Verification items for the finished model (mm, model axes). Face numbers are marked on the shaded views. A direction names the side the tool comes from. Coordinates: 2 decimals unless noted, no trailing zeros. Write each loop counter-clockwise with the first axis right and the second up, starting at its lowest first coordinate (ties: lowest second). Pieces come first, ordered by that corner, then holes. Notation, with made-up numbers: (33.5, -1.5) - (75.5, -1.5) arc R22 cw to (75.5, 19.5) - close; hole circle Ø2 at (57, 58.25). An arc over 180 degrees is marked (long way). Answer as CSV lines item,"result". Start each with the question number.
```python
from build123d import *

# Parameters (mm, degrees)
ESQUISSE1_W              = 8.5
ESQUISSE1_H              = 72
ESQUISSE1_R              = 2.1
BOSS_EXTRU_1_DEPTH       = 17.5
ENL_V_START              = -3
ENL_V_MAT_EXTRU_4_DEPTH  = 3.5
ESQUISSE7_R              = 2.1
BOSS_EXTRU_3_DEPTH       = 7
ESQUISSE3_W              = 8.5
ESQUISSE3_H              = 4
ENL_V_MAT_EXTRU_3_DEPTH  = 19
BOSS_EXTRU_2_START       = -7
BOSS_EXTRU_2_DEPTH       = 12
ESQUISSE8_W              = 8.5
ESQUISSE8_H              = 7
BOSS_EXTRU_4_DEPTH       = 4
ESQUISSE9_R              = 1.6
ENL_V_MAT_EXTRU_5_DEPTH  = 5
ENL_V_START_2            = -4
ESQUISSE10_R             = 1.6
ENL_V_MAT_EXTRU_6_DEPTH  = 2.6
ESQUISSE11_R             = 1.6
ENL_V_MAT_EXTRU_7_DEPTH  = 1.6
ESQUISSE14_W             = 2.5
ESQUISSE14_H             = 10
ENL_V_MAT_EXTRU_9_DEPTH  = 17.6
CHANFREIN1_SIZE          = 0.5
ESQUISSE15_W             = 8.5
ESQUISSE15_H             = 15
ESQUISSE15_W_2           = 2.6
ESQUISSE15_H_2           = 5.7
ESQUISSE15_W_3           = 2.5
ESQUISSE15_H_3           = 10
ENL_V_MAT_EXTRU_10_DEPTH = 10
CHANFREIN2_SIZE          = 9


with BuildPart() as part:
    # Esquisse1 → Boss.-Extru.1 (new body)
    with BuildSketch(Plane.XY):
        with Locations((4.25, 36)):
            Rectangle(ESQUISSE1_W, ESQUISSE1_H)
        with Locations((4, 20.5)):
            Circle(ESQUISSE1_R, mode=Mode.SUBTRACT)
        with Locations((4, 51.5)):
            Circle(ESQUISSE1_R, mode=Mode.SUBTRACT)
    extrude(amount=BOSS_EXTRU_1_DEPTH)

    # Esquisse6 → Enlèv. mat.-Extru.4 (cut)
    with BuildSketch(Plane.XY.offset(17.5).offset(ENL_V_START)):
        Polygon((7.55, 22.549593456), (4, 24.599186911), (0.45, 22.549593456), (0.45, 18.450406544), (4, 16.400813089), (7.55, 18.450406544), align=None)
        Polygon((8.5, 24.599186911), (4, 24.599186911), (7.55, 22.549593456), (7.55, 18.450406544), (4, 16.400813089), (8.5, 16.400813089), align=None)
    enl_v_mat_extru_4 = extrude(amount=-ENL_V_MAT_EXTRU_4_DEPTH, mode=Mode.SUBTRACT)

    # Esquisse7 → Boss.-Extru.3 (add)
    with BuildSketch(Plane(origin=(0, 0, 0), x_dir=(-1, 0, 0), z_dir=(0, 0, -1))):
        with Locations((-4, 20.5)):
            Circle(ESQUISSE7_R)
    boss_extru_3 = extrude(amount=-BOSS_EXTRU_3_DEPTH)

    # Esquisse3 → Enlèv. mat.-Extru.3 (cut)
    with BuildSketch(Plane(origin=(0, 0, 0), x_dir=(-1, 0, 0), z_dir=(0, -1, 0))):
        with Locations((-4.25, -2)):
            Rectangle(ESQUISSE3_W, ESQUISSE3_H)
    enl_v_mat_extru_3 = extrude(amount=-ENL_V_MAT_EXTRU_3_DEPTH, mode=Mode.SUBTRACT)

    # Esquisse5 → Boss.-Extru.2 (add)
    with BuildSketch(Plane.XZ.offset(BOSS_EXTRU_2_START)):
        with BuildLine():
            ThreePointArc((4.662966644, 1.130359715), (4.682946936, 1.236721088), (4.714353535, 1.340285461))
            ThreePointArc((4.714353535, 1.340285461), (5.229781903, 1.749631615), (5.773646598, 1.378900082))
            ThreePointArc((5.773646598, 1.378900082), (5.814751932, 1.256791784), (5.839789089, 1.130406557))
            ThreePointArc((5.839789089, 1.130406557), (5.889607538, 1.037219203), (5.988503907, 1))
            Line((5.988503907, 1), (6.514258005, 1))
            ThreePointArc((6.514258005, 1), (6.613136611, 1.037203629), (6.662966644, 1.130359715))
            ThreePointArc((6.662966644, 1.130359715), (6.682946936, 1.236721088), (6.714353535, 1.340285461))
            ThreePointArc((6.714353535, 1.340285461), (7.229781903, 1.749631615), (7.773646598, 1.378900082))
            ThreePointArc((7.773646598, 1.378900082), (7.814751933, 1.256791779), (7.83978909, 1.130406547))
            ThreePointArc((7.83978909, 1.130406547), (7.889607542, 1.037219199), (7.988503907, 1))
            Line((7.988503907, 1), (8.5, 1))
            Line((8.5, 1), (8.5, 4))
            Line((8.5, 4), (0, 4))
            Line((0, 4), (0, 1))
            Line((0, 1), (0.514258005, 1))
            ThreePointArc((0.514258005, 1), (0.613136611, 1.037203629), (0.662966644, 1.130359715))
            ThreePointArc((0.662966644, 1.130359715), (0.682946936, 1.236721088), (0.714353535, 1.340285461))
            ThreePointArc((0.714353535, 1.340285461), (1.229781903, 1.749631615), (1.773646598, 1.378900082))
            ThreePointArc((1.773646598, 1.378900082), (1.814751933, 1.256791781), (1.83978909, 1.130406551))
            ThreePointArc((1.83978909, 1.130406551), (1.88960754, 1.037219201), (1.988503907, 1))
            Line((1.988503907, 1), (2.514258005, 1))
            ThreePointArc((2.514258005, 1), (2.613136611, 1.037203629), (2.662966644, 1.130359715))
            ThreePointArc((2.662966644, 1.130359715), (2.682946936, 1.236721088), (2.714353535, 1.340285461))
            ThreePointArc((2.714353535, 1.340285461), (3.229781903, 1.749631615), (3.773646598, 1.378900082))
            ThreePointArc((3.773646598, 1.378900082), (3.814751933, 1.256791781), (3.83978909, 1.130406551))
            ThreePointArc((3.83978909, 1.130406551), (3.88960754, 1.037219201), (3.988503907, 1))
            Line((3.988503907, 1), (4.514258005, 1))
            ThreePointArc((4.514258005, 1), (4.613136611, 1.037203629), (4.662966644, 1.130359715))
        make_face()
    boss_extru_2 = extrude(amount=-BOSS_EXTRU_2_DEPTH)

    # Esquisse8 → Boss.-Extru.4 (add)
    with BuildSketch(Plane(origin=(0, 0, 4), x_dir=(-1, 0, 0), z_dir=(0, 0, -1))):
        with Locations((-4.25, 3.5)):
            Rectangle(ESQUISSE8_W, ESQUISSE8_H)
    boss_extru_4 = extrude(amount=BOSS_EXTRU_4_DEPTH)

    # Esquisse9 → Enlèv. mat.-Extru.5 (cut)
    with BuildSketch(Plane(origin=(0, 0, 0), x_dir=(-1, 0, 0), z_dir=(0, 0, -1))):
        with Locations((-4.25, 3.75)):
            Circle(ESQUISSE9_R)
        with Locations((-4.25, 22.25)):
            Circle(ESQUISSE9_R)
    enl_v_mat_extru_5 = extrude(amount=-ENL_V_MAT_EXTRU_5_DEPTH, mode=Mode.SUBTRACT)

    # Esquisse10 → Enlèv. mat.-Extru.6 (cut)
    # profile 1 of 4: a face of its own
    with BuildSketch(Plane(origin=(0, 0, 0), x_dir=(-1, 0, 0), z_dir=(0, 0, -1)).offset(ENL_V_START_2)):
        Polygon((-2.604551733, 25.1), (-5.895448267, 25.1), (-7.540896534, 22.25), (-5.895448267, 19.4), (-2.604551733, 19.4), (-0.959103466, 22.25), align=None)
        with Locations((-4.25, 22.25)):
            Circle(ESQUISSE10_R, mode=Mode.SUBTRACT)
    # profile 2 of 4: a face of its own
    with BuildSketch(Plane(origin=(0, 0, 0), x_dir=(-1, 0, 0), z_dir=(0, 0, -1)).offset(ENL_V_START_2)):
        Polygon((-2.604551733, 6.6), (-5.895448267, 6.6), (-7.540896534, 3.75), (-5.895448267, 0.9), (-2.604551733, 0.9), (-0.959103466, 3.75), align=None)
    # profile 3 of 4: a face of its own
    with BuildSketch(Plane(origin=(0, 0, 0), x_dir=(-1, 0, 0), z_dir=(0, 0, -1)).offset(ENL_V_START_2)):
        Polygon((-8.5, 6.6), (-5.895448267, 6.6), (-7.540896534, 3.75), (-5.895448267, 0.9), (-8.5, 0.9), align=None)
    # profile 4 of 4: a face of its own
    with BuildSketch(Plane(origin=(0, 0, 0), x_dir=(-1, 0, 0), z_dir=(0, 0, -1)).offset(ENL_V_START_2)):
        Polygon((-7.540896534, 22.25), (-5.895448267, 25.1), (-8.5, 25.1), (-8.5, 19.4), (-5.895448267, 19.4), align=None)
    enl_v_mat_extru_6 = extrude(amount=-ENL_V_MAT_EXTRU_6_DEPTH, mode=Mode.SUBTRACT)

    # Esquisse11 → Enlèv. mat.-Extru.7 (cut)
    with BuildSketch(Plane(origin=(0, 0, 5), x_dir=(-1, 0, 0), z_dir=(0, 0, -1))):
        with Locations((-4.25, 22.25)):
            Circle(ESQUISSE11_R)
    enl_v_mat_extru_7 = extrude(amount=-ENL_V_MAT_EXTRU_7_DEPTH, mode=Mode.SUBTRACT)

    # Esquisse14 → Enlèv. mat.-Extru.9 (cut)
    with BuildSketch(Plane(origin=(8.5, 0, 0), x_dir=(0, 0, -1), z_dir=(1, 0, 0))):
        with Locations((-6.75, 13)):
            Rectangle(ESQUISSE14_W, ESQUISSE14_H)
    enl_v_mat_extru_9 = extrude(amount=-ENL_V_MAT_EXTRU_9_DEPTH, mode=Mode.SUBTRACT)

    # Symétrie14: Enlèv. mat.-Extru.4, Boss.-Extru.3, Enlèv. mat.-Extru.3, Boss.-Extru.2, Boss.-Extru.4, Enlèv. mat.-Extru.5, Enlèv. mat.-Extru.6, Enlèv. mat.-Extru.7, Enlèv. mat.-Extru.9 across plane
    add(enl_v_mat_extru_4.mirror(Plane(origin=(0, 36, 0), x_dir=(0, 0, 1), z_dir=(0, -1, 0))), mode=Mode.SUBTRACT)
    add(boss_extru_3.mirror(Plane(origin=(0, 36, 0), x_dir=(0, 0, 1), z_dir=(0, -1, 0))))
    add(enl_v_mat_extru_3.mirror(Plane(origin=(0, 36, 0), x_dir=(0, 0, 1), z_dir=(0, -1, 0))), mode=Mode.SUBTRACT)
    add(boss_extru_2.mirror(Plane(origin=(0, 36, 0), x_dir=(0, 0, 1), z_dir=(0, -1, 0))))
    add(boss_extru_4.mirror(Plane(origin=(0, 36, 0), x_dir=(0, 0, 1), z_dir=(0, -1, 0))))
    add(enl_v_mat_extru_5.mirror(Plane(origin=(0, 36, 0), x_dir=(0, 0, 1), z_dir=(0, -1, 0))), mode=Mode.SUBTRACT)
    add(enl_v_mat_extru_6.mirror(Plane(origin=(0, 36, 0), x_dir=(0, 0, 1), z_dir=(0, -1, 0))), mode=Mode.SUBTRACT)
    add(enl_v_mat_extru_7.mirror(Plane(origin=(0, 36, 0), x_dir=(0, 0, 1), z_dir=(0, -1, 0))), mode=Mode.SUBTRACT)
    add(enl_v_mat_extru_9.mirror(Plane(origin=(0, 36, 0), x_dir=(0, 0, 1), z_dir=(0, -1, 0))), mode=Mode.SUBTRACT)

    # Chanfrein1
    chanfrein1_edges = [part.edges().sort_by_distance(p)[0] for p in [
        (1.9, 51.5, 14.5),
        (1.9, 51.5, 11),
        (1.9, 20.5, 11),
        (1.9, 20.5, 14.5),
    ]]
    chamfer(chanfrein1_edges, length=CHANFREIN1_SIZE)

    # Esquisse15 → Enlèv. mat.-Extru.10 (cut)
    # profile 1 of 2: a face of its own
    with BuildSketch(Plane(origin=(8.5, 0, 0), x_dir=(0, 0, -1), z_dir=(1, 0, 0))):
        with Locations((-13.25, 7.5)):
            Rectangle(ESQUISSE15_W, ESQUISSE15_H)
    # profile 2 of 2: a face of its own
    with BuildSketch(Plane(origin=(8.5, 0, 0), x_dir=(0, 0, -1), z_dir=(1, 0, 0))):
        Polygon((-9, 0), (0, 0), (0, 7), (-1, 7), (-1, 19), (0, 19), (0, 46), (-9, 46), (-9, 15), align=None)
        with Locations((-5.3, 3.75)):
            Rectangle(ESQUISSE15_W_2, ESQUISSE15_H_2, mode=Mode.SUBTRACT)
        with Locations((-6.75, 13)):
            Rectangle(ESQUISSE15_W_3, ESQUISSE15_H_3, mode=Mode.SUBTRACT)
        with Locations((-5.3, 22.25)):
            Rectangle(ESQUISSE15_W_2, ESQUISSE15_H_2, mode=Mode.SUBTRACT)
    extrude(amount=-ENL_V_MAT_EXTRU_10_DEPTH, mode=Mode.SUBTRACT)


with BuildPart() as enl_v_mat_extru_10_kept_piece:
    # of the separate pieces the step leaves, the one the design keeps (enl_v_mat_extru_10_pieces_kept)
    add(part.part.solids().sort_by_distance((6.6, 20.5, 14.5))[0])

    # Chanfrein2
    chanfrein2_edges = [enl_v_mat_extru_10_kept_piece.edges().sort_by_distance(p)[0] for p in [
        (4.25, 46, 9),
    ]]
    chamfer(chanfrein2_edges, length=CHANFREIN2_SIZE - 0.0001)  # a hair under: the kernel refuses the full size


solid = enl_v_mat_extru_10_kept_piece.part
```
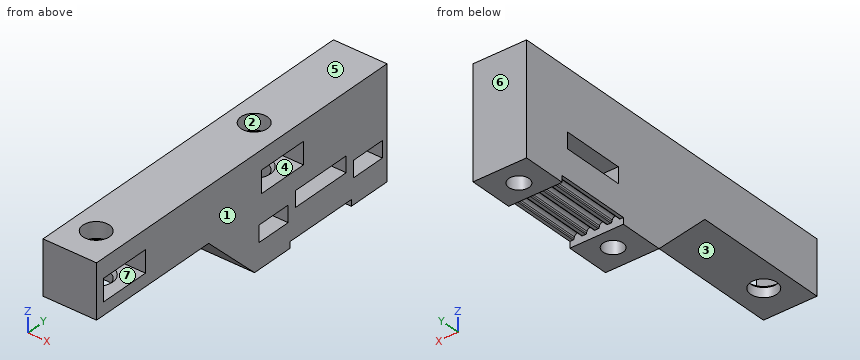
1. Draft check along Y on the marked faces 5, 6 and 7. Enter one of: pulls with the +Y half, pulls with the -Y half, needs draft (parallel to the pull), parting line crosses it, or undercut.
2. Scan lines: line 1 along Y through (x, z) = (4.25, 11.25); line 2 along Y through (x, z) = (4, 9.75); line 3 along Z through (x, y) = (4.25, 24). Record each from-to range of solid material in increasing order. Write a range as from..to.
3. Access from +Z, -Z, +X, -X, +Y, -Y to the whole of each face (thin tool, end or side, straight path). Record for the marked faces 1, 2, 3 and 4.
4. Depth check by flat-ended pin: P1, Ø1.8, axis at y = 21, z = 13, coming from the +X side; P2, Ø5, axis at x = 4, y = 20.5, coming from the -Z side; P3, Ø2, axis at x = 7, y = 57.5, coming from the -Z side; P4, Ø6, axis at y = 31, z = 4.5, coming from the +X side. Enter the tip coordinate at first touch or a pass-through.
5. Cross-section at C-C (z = 15.5). Record the cut outline in (x, y), and give its area (3 significant figures).
6. Cross-section at D-D (y = 32). Record the cut outline in (x, z), and give its area (4 significant figures).
7. Cross-section at A-A (y = 20.5). Record the cut outline in (x, z).
Completed:
1,face 5,"needs draft"
1,face 6,"pulls with the +Y half"
1,face 7,"undercut"
2,line 1,"y = 15..16.4, 24.6..47.4, 55.6..72"
2,line 2,"y = 15..18.4, 22.6..49.4, 53.6..72"
2,line 3,"z = 9..11, 14.5..17.5"
3,face 1,"+Z, -Z, +X, +Y, -Y"
3,face 2,"+Z"
3,face 3,"-Z, +X, -X, -Y"
3,face 4,"+X"
4,P1,"stops at x = 0.45"
4,P2,"stops at z = 9"
4,P3,"stops at z = 1"
4,P4,"passes through"
5,outline,"(0, 15) - (8.5, 15) - (8.5, 72) - (0, 72) - close; hole circle Ø4.2 at (4, 20.5); hole circle Ø4.2 at (4, 51.5)"
5,area,"457 mm2"
6,outline,"(0, 9) - (8.5, 9) - (8.5, 17.5) - (0, 17.5) - close"
6,area,"72.25 mm2"
7,outline,"(0, 9) - (1.9, 9) - (1.9, 10.5) - (1.4, 11) - (0.45, 11) - (0.45, 14.5) - (1.4, 14.5) - (1.9, 15) - (1.9, 17.5) - (0, 17.5) - close; (6.1, 9) - (8.5, 9) - (8.5, 11) - (6.6, 11) - (6.1, 10.5) - close; (6.1, 15) - (6.6, 14.5) - (8.5, 14.5) - (8.5, 17.5) - (6.1, 17.5) - close"
